Design review of the part built by this model. Coordinates are the model's own, in mm. A direction names the side the tool comes from. Give positions to 0.01 mm unless a question says otherwise; leave off trailing zeros. Order: outer loops, then holes, each group sorted by start corner. A loop starts at its lowest first (then second) coordinate and runs counter-clockwise, first axis right, second up. Notation, with made-up numbers: (75.25, 89.5) - (116.25, 89.5) arc R23 ccw to (116.25, 113.5) - close; hole circle Ø1 at (-32, -9.75). An arc over 180 degrees is marked (long way). Write each question's results on one line, items separated by ' | '. Start each with the question number.
```python
from build123d import *

# Parameters (mm, degrees)
F0_W     = 12.7
F0_H     = 88.9
F1_DEPTH = 12.7
F2_W     = 12.7
F2_H     = 10.96398
F3_DEPTH = 30.734
F4_W     = 12.7
F4_H     = 12.7
F5_DEPTH = 25.4
F6_W     = 12.7
F6_H     = 10.96398
F7_DEPTH = 16.51
F8_W     = 12.7
F8_H     = 12.7
F9_DEPTH = 31.242


with BuildPart() as f1:
    # F0 (on Front) → F1 (new body)
    with BuildSketch(Plane.XZ):
        with Locations((-31.999755, -44.45)):
            Rectangle(F0_W, F0_H)
    extrude(amount=F1_DEPTH)

    # F2 (on face) → F3 (join)
    with BuildSketch(Plane.XZ.offset(12.7)):
        with Locations((-31.999755, -18.141449)):
            Rectangle(F2_W, F2_H)
    extrude(amount=F3_DEPTH)

    # F4 (on face) → F5 (join)
    with BuildSketch(Plane.XY):
        with Locations((-31.999755, -6.35)):
            Rectangle(F4_W, F4_H)
    extrude(amount=F5_DEPTH)

    # F6 (on face) → F7 (join)
    with BuildSketch(Plane.XZ.offset(43.434)):
        with Locations((-31.999755, -18.141449)):
            Rectangle(F6_W, F6_H)
    extrude(amount=F7_DEPTH)

    # F8 (on face) → F9 (join)
    with BuildSketch(Plane.XY.offset(-12.659459)):
        with Locations((-31.999755, -53.594)):
            Rectangle(F8_W, F8_H)
    extrude(amount=F9_DEPTH)


solid = f1.part
```
Q1. Add section A-A (x = -33.5). Give the boundary of the cut face in (y, z), plus the area to 3 significant figures.
Q2. Draft analysis for pull direction Y (two halves, no side actions). For faces 1 (the flat face through (-32, 0, -33)), 2 (the flat face through (-32, -54, 18.583)), 3 (the flat face through (-32, -30, -12.659)), state which applies: pulls with the +Y half, pulls with the -Y half, needs draft (parallel to the pull), parting line crosses it, or undercut.
Q3. Machinability: for faces 4 (the flat face through (-32, -12.7, -56)), 5 (the flat face through (-32, -12.7, 6)), 6 (the flat face through (-32, -6, -88.9)), which of the approach directions +Z, -Z, +X, -X, +Y, -Y give a long, thin tool a straight path to every point of the face, cutting with its end or side? Answer none if there is none.
Q4. For line 1 (Y direction, x = -31.25, z = -7); line 2 (Z direction, x = -28.25, y = -56.5); line 3 (Z direction, x = -34.5, y = -37), list the stretches that pass through material, from the lowest coordinate up. Write a range as [from, to].
Q5. Insertion check: pin 1 Ø5 at (x, y) = (-28, -50) entering from +Z; pin 2 Ø5 at (x, y) = (-37, -41.5) entering from +Z. Each pin has a flat end and moves straight along its axis. Give the tip position at first contact, or say it passes through.
Q6. Add section C-C (y = -50). Give the boundary of the cut face in (x, z), plus the area to 3 significant figures.
Q7. Add section B-B (z = -75). Give the boundary of the cut face in (x, y).
Verdict:
1) outline: (-59.94, -23.62) - (-12.7, -23.62) - (-12.7, -88.9) - (0, -88.9) - (0, 25.4) - (-12.7, 25.4) - (-12.7, -12.66) - (-47.24, -12.66) - (-47.24, 18.58) - (-59.94, 18.58) - close | area: 2,370 mm2
2) face 1: pulls with the +Y half | face 2: needs draft | face 3: undercut
3) face 4: -Z, +X, -X, -Y | face 5: +Z, +X, -X | face 6: -Z, +X, -X, +Y, -Y
4) line 1: y = [-59.94, -47.24], [-12.7, 0] | line 2: z = [-23.62, 18.58] | line 3: z = [-23.62, -12.66]
5) pin 1: stops at z = 18.58 | pin 2: stops at z = -12.66
6) outline: (-38.35, -23.62) - (-25.65, -23.62) - (-25.65, 18.58) - (-38.35, 18.58) - close | area: 536 mm2
7) outline: (-38.35, -12.7) - (-25.65, -12.7) - (-25.65, 0) - (-38.35, 0) - close
